Design review of the part built by this model. Coordinates are the model's own, in mm. A direction names the side the tool comes from. Give positions to 0.01 mm unless a question says otherwise; leave off trailing zeros. Loops run counter-clockwise (first coordinate to the right, second up) from the corner with the lowest first, then second, coordinate; pieces in that order, holes last. Notation, with made-up numbers: (61, 4.25) -> (87, 4.25) arc R36 ccw to (87, 43.25) -> close; hole circle Ø9 at (-7, 2). An arc over 180 degrees is marked (long way). Use CSV: the item, a comma, the result in double quotes. Start each with the question number.
Item 1: The part is to be moulded in two halves that separate along X. For faces 1 (the face through (-1.73, -7.81, 21.26)), 2 (the face through (9, 0, 0)), 3 (the face through (6, 0, 1)), 4 (the face through (8, -0.1, 0.5)), say which applies: +X half, -X half, draft (parallel to the pull), parting line (faces both ways), or undercut.
Item 2: Wall thickness on line 1 along Z through (x, y) = (-6.5, 6); line 2 along Y through (x, z) = (-0.25, 32.5); line 3 along X through (y, z) = (-5.5, 24): over which ranges is each line inside the solid? List them lowest first. Write a range as from..to.
Item 3: Clearance check with flat-ended pins moving along their axes: pin 1 (1.5 mm diameter, centred on x = 6, y = 4.5, fed in from -Z); pin 2 (5 mm diameter, centred on y = -6, z = 21.5, fed in from -X); pin 3 (8 mm diameter, centred on x = 0, z = 37, fed in from +Y). State where each tip first meets the part, or that it passes through.
Item 4: For faces 5 (the face through (4, -0.1, 0.5)), 6 (the face through (-2, 0, 0)), 7 (the face through (-2.681, 6.466, 41.535)), list the 3-axis set-ups (+Z, -Z, +X, -X, +Y, -Y) from which the entire face can be reached by the end or side of a thin tool; tool diameter is ignored.
Item 5: We need section C-C (z = 3.5). State the section outline as (x, y) points, plus the area to 3 significant figures.
Item 6: We need section A-A (y = 0). State the section outline as (x, z) points, plus the area to 3 significant figures.
Item 7: We need section B-B (x = 0). State the section outline as (y, z) points, plus the area to 3 significant figures.
Item 8: We need section D-D (x = 6.5). State the section outline as (y, z) points, plus the area to 3 significant figures.
from build123d import *

# Parameters (mm, degrees)
F0_R     = 10.5
F1_DEPTH = 4
F2_R     = 8
F3_DEPTH = 39
F4_W     = 7
F4_H     = 5
F6_W     = 4
F6_H     = 24.978078
F7_DEPTH = 1


with BuildPart() as f1:
    # F0 (on Top) → F1 (new body)
    with BuildSketch(Plane.XY):
        Circle(F0_R)
    extrude(amount=F1_DEPTH)

    # F2 (on Top) → F3 (join)
    with BuildSketch(Plane.XY):
        Circle(F2_R)
    extrude(amount=F3_DEPTH)

    # F4 (on Right) → F5 (revolve)
    with BuildSketch(Plane.YZ):
        with Locations((3.5, 41.5)):
            Rectangle(F4_W, F4_H)
    revolve(axis=Axis((0, 0, 41.5), (0, 0, -1)))

    # F6 (on Top) → F7 (cut)
    with BuildSketch(Plane.XY):
        with Locations((6, 1.013985)):
            Rectangle(F6_W, F6_H)
    extrude(amount=F7_DEPTH, mode=Mode.SUBTRACT)


solid = f1.part
Results found:
1,face 1,"parting line"
1,face 2,"draft"
1,face 3,"undercut"
1,face 4,"undercut"
2,line 1,"0..4"
2,line 2,"-8..8"
2,line 3,"-5.81..5.81"
3,pin 1,"z = 1"
3,pin 2,"x = -7.19"
3,pin 3,"y = 8"
4,face 5,"-Z, +Y, -Y"
4,face 6,"-Z, +X, -X, +Y, -Y"
4,face 7,"+Z"
5,outline,"circle Ø21 at (0, 0)"
5,area,"346 mm²"
6,outline,"(-10.5, 0) -> (4, 0) -> (4, 1) -> (8, 1) -> (8, 0) -> (10.5, 0) -> (10.5, 4) -> (8, 4) -> (8, 39) -> (7, 39) -> (7, 44) -> (-7, 44) -> (-7, 39) -> (-8, 39) -> (-8, 4) -> (-10.5, 4) -> close"
6,area,"710 mm²"
7,outline,"(-10.5, 0) -> (10.5, 0) -> (10.5, 4) -> (8, 4) -> (8, 39) -> (7, 39) -> (7, 44) -> (-7, 44) -> (-7, 39) -> (-8, 39) -> (-8, 4) -> (-10.5, 4) -> close"
7,area,"714 mm²"
8,outline,"(-8.25, 1) -> (8.25, 1) -> (8.25, 4) -> (4.66, 4) -> (4.66, 39) -> (2.6, 39) -> (2.6, 44) -> (-2.6, 44) -> (-2.6, 39) -> (-4.66, 39) -> (-4.66, 4) -> (-8.25, 4) -> close"
8,area,"402 mm²"
